Model file for the job. Use its own axes, mm. Face numbers are marked on the shaded views. Round coordinates to 2 decimals unless told otherwise and drop trailing zeros. Loops run counter-clockwise (first coordinate to the right, second up) from the corner with the lowest first, then second, coordinate; pieces in that order, holes last. Notation, with made-up numbers: M 86,-7 L 132,-7 A24 ccw 132,17 Z; hole C 71.25,-15 d10. An arc over 180 degrees is marked long. Use a Markdown table: item, result. Add a question column.
Item 1: Wall check: L1, parallel to Y at x = 0, z = 9.75; L2, parallel to Y at x = 17, z = 6.75; L3, parallel to Z at x = -5.5, y = 1. Give the ranges that are in metal, low to high. Write a range as from..to.
Item 2: Saw through at C-C on y = 0. Write the cut outline in (x, z).
Item 3: Saw through at A-A on z = 6. Write the cut outline in (x, y), then the cut area to 3 significant figures.
Item 4: Saw through at D-D on x = 0. Write the cut outline in (y, z), then the cut area to 3 significant figures.
Item 5: Two-plate mould, pull along Y, no slides. Class the marked faces 1, 2 and 3: +Y half, -Y half, draft (parallel to the pull), parting line (faces both ways), or undercut.
Item 6: Pin check, flat tips, straight feed: P1, Ø8, axis at x = -3, z = 3, coming from the -Y side; P2, Ø6, axis at x = -8.5, y = 10, coming from the +Z side; P3, Ø12, axis at x = -5.5, y = -4.5, coming from the +Z side. Stop position of each tip, or through.
Item 7: Saw through at B-B on y = 11. Write the cut outline in (x, z).
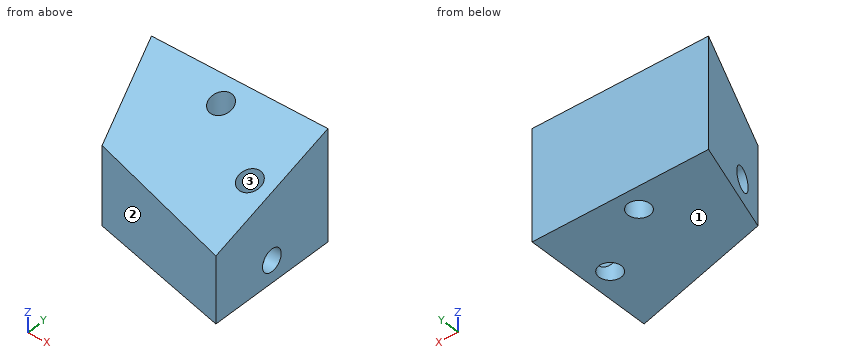
```python
from build123d import *

# Parameters (mm, degrees)
F0_R     = 2.5
F1_DEPTH = 25
F2_R     = 2.5
F3_DEPTH = 40.001


with BuildPart() as f1:
    # F0 (on Top) → F1 (new body)
    with BuildSketch(Plane.XY):
        Polygon((20, -15), (20, 15), (-20, 15), (-12.727273, -6.818182), align=None)
        with Locations((15, 0)):
            Circle(F0_R, mode=Mode.SUBTRACT)
        with Locations((0, 10)):
            Circle(F0_R, mode=Mode.SUBTRACT)
    extrude(amount=F1_DEPTH)

    # F2 (on face) → F3 (cut, through all)
    with BuildSketch(Plane.YZ.offset(20)):
        with Locations((0, 5)):
            Circle(F2_R)
        Polygon((-15, 15), (15, 25), (-15, 25), align=None)
    extrude(amount=-F3_DEPTH, mode=Mode.SUBTRACT)


solid = f1.part
```
Entries:
| question | item | result |
|---|---|---|
| 1 | L1 | -10..7.5, 12.5..15 |
| 1 | L2 | -14.25..-1.79, 1.79..15 |
| 1 | L3 | 0..2.71, 7.29..20.33 |
| 2 | outline | M -15,0 L 12.5,0 L 12.5,2.5 L -15,2.5 Z; M -15,7.5 L 12.5,7.5 L 12.5,20 L -15,20 Z; M 17.5,0 L 20,0 L 20,2.5 L 17.5,2.5 Z; M 17.5,7.5 L 20,7.5 L 20,20 L 17.5,20 Z |
| 3 | outline | M -20,15 L -15.76,2.29 L 14,2.29 A2.5 cw 16,2.29 L 20,2.29 L 20,15 Z; M -14.24,-2.29 L -12.73,-6.82 L 20,-15 L 20,-2.29 L 16,-2.29 A2.5 cw 14,-2.29 Z; hole C 0,10 d5 |
| 3 | area | 747 mm2 |
| 4 | outline | M -10,0 L 7.5,0 L 7.5,22.5 L -10,16.67 Z; M 12.5,0 L 15,0 L 15,25 L 12.5,24.17 Z; hole C 0,5 d5 |
| 4 | area | 385 mm2 |
| 5 | face 1 | draft |
| 5 | face 2 | -Y half |
| 5 | face 3 | undercut |
| 6 | P1 | y = -10.25 |
| 6 | P2 | z = 24.33 |
| 6 | P3 | z = 20.5 |
| 7 | outline | M -18.67,0 L -2.29,0 L -2.29,23.67 L -18.67,23.67 Z; M 2.29,0 L 20,0 L 20,23.67 L 2.29,23.67 Z |
